```python
from build123d import *

# Parameters (mm, degrees)
EXTRUDE_THIN1_DEPTH = 317.5
FILLET1_R           = 1.016


with BuildPart() as part:
    # Sketch1 → Extrude-Thin1 (new body)
    with BuildSketch(Plane.XY):
        with BuildLine():
            Line((0, 6.35), (0, 0))
            Line((0, 0), (-3.96875, 0))
            Line((-3.96875, 0), (-3.96875, 4.7625))
            Line((-3.96875, 4.7625), (-6.35, 4.7625))
            ThreePointArc((-6.35, 4.7625), (-8.34834139, 13.302516912), (-14.576333586, 19.478063073))
            ThreePointArc((-14.576333586, 19.478063073), (-17.085021571, 22.337680243), (-17.166208015, 26.140880807))
            ThreePointArc((-17.166208015, 26.140880807), (-15.447363075, 28.466364673), (-12.7, 29.36875))
            Line((-12.7, 29.36875), (-12.7, 31.75))
            Line((-12.7, 31.75), (0, 30.1625))
            Line((0, 30.1625), (0, 26.9875))
            Line((0, 26.9875), (-1.016, 26.9875))
            Line((-1.016, 26.9875), (-1.016, 29.265593266))
            Line((-1.016, 29.265593266), (-11.684, 30.599093266))
            Line((-11.684, 30.599093266), (-11.684, 28.224203151))
            ThreePointArc((-11.684, 28.224203151), (-14.420615811, 27.912235037), (-16.204387121, 25.813533029))
            ThreePointArc((-16.204387121, 25.813533029), (-16.138046198, 22.705774854), (-14.08808973, 20.369059109))
            ThreePointArc((-14.08808973, 20.369059109), (-7.729180549, 14.259833631), (-5.315606066, 5.7785))
            Line((-5.315606066, 5.7785), (-2.95275, 5.7785))
            Line((-2.95275, 5.7785), (-2.95275, 1.016))
            Line((-2.95275, 1.016), (-1.016, 1.016))
            Line((-1.016, 1.016), (-1.016, 6.35))
            Line((-1.016, 6.35), (0, 6.35))
        make_face()
    extrude(amount=-EXTRUDE_THIN1_DEPTH)

    # Fillet1
    fillet1_edges = [part.edges().sort_by_distance(p)[0] for p in [
        (-11.684, 28.224203151, -158.75),
        (-2.95275, 5.7785, -158.75),
        (0, 0, -158.75),
        (-3.96875, 0, -158.75),
        (-6.35, 4.7625, -158.75),
        (-12.7, 31.75, -158.75),
        (0, 30.1625, -158.75),
    ]]
    fillet(fillet1_edges, radius=FILLET1_R)


solid = part.part
```
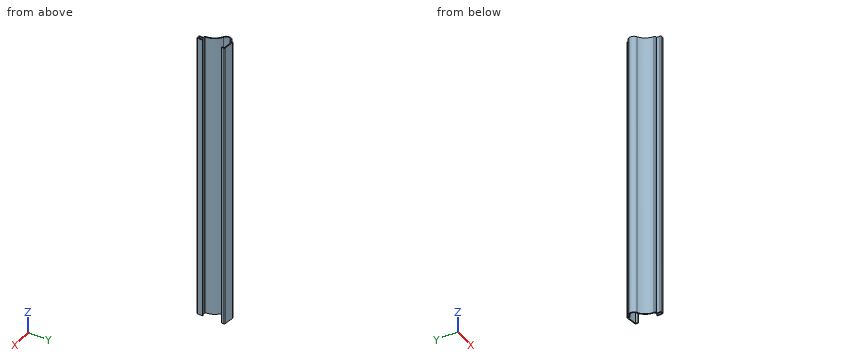
Geometry: final body of the model. Coordinates: model frame, mm. Give positions to 0.01 mm unless a question says otherwise; leave off trailing zeros. Order: outer loops, then holes, each group sorted by start corner. A loop starts at its lowest first (then second) coordinate and runs counter-clockwise, first axis right, second up. Notation, with made-up numbers: (74, -18) -> (112, -18) arc R20 ccw to (112, -2) -> close; hole circle Ø9 at (-35, -36). An arc over 180 degrees is marked (long way). Write each question's results on one line, items separated by ' | '. Start each with the question number.
1) Section C-C (y = 10). Return loops of the section in (x, z).
2) First-contact query: pin 1 (1.1 mm diameter, centred on y = 28, z = -121, fed in from -X); pin 2 (0.7 mm diameter, centred on x = -4.5, z = -137.5, fed in from +Y); pin 3 (6 mm diameter, centred on y = 3, z = -203.5, fed in from -X); pin 4 (1.9 mm diameter, centred on y = 2, z = -233.5, fed in from +X). Flat tips, straight axial feed; report the tip coordinate or a pass-through.
3) Line query: line 1 (Y direction, x = -16, z = -223); line 2 (Y direction, x = -4, z = -61); line 3 (X direction, y = 5, z = -145.5). Output: solid intervals per line, ascending. Write a range as from..to.
4) Section B-B (x = -9). Return loops of the section in (y, z), then the cut area to 3 significant figures.
Calculated:
1) outline: (-6.96, -317.5) -> (-5.91, -317.5) -> (-5.91, 0) -> (-6.96, 0) -> close
2) pin 1: x = -16.48 | pin 2: y = 30.77 | pin 3: x = -6.34 | pin 4: x = 0
3) line 1: 20.59..22.39, 26.3..28 | line 2: 4.76..5.78, 29.64..30.66 | line 3: -5.97..-2.98, -1.02..0
4) outline: (14.37, -317.5) -> (16.09, -317.5) -> (16.09, 0) -> (14.37, 0) -> close; (30.26, -317.5) -> (31.29, -317.5) -> (31.29, 0) -> (30.26, 0) -> close | area: 872 mm2
